The model under review builds one solid part; all positions refer to its coordinate system, in mm. A direction names the side the tool comes from. Round coordinates to 2 decimals unless told otherwise and drop trailing zeros. Write each loop counter-clockwise with the first axis right and the second up, starting at its lowest first coordinate (ties: lowest second). Pieces come first, ordered by that corner, then holes. Notation, with made-up numbers: M 56,-0.75 L 78,-0.75 A12 ccw 78,7.25 Z; hole C -1.75,52.25 d1. An arc over 180 degrees is marked long. One line per item, written item: value. Start each with the question number.
1) For P1, Ø2, axis at x = -1, z = 6, coming from the +Y side; P2, Ø1.5, axis at x = 12, z = 5, coming from the -Y side; P3, Ø2, axis at x = 5.5, z = 4, coming from the +Y side; P4, Ø3, axis at y = 6, z = 5.5, coming from the +X side, all flat-tipped, find the tip position at first contact; note any pin that passes through.
2) Take a section at D-D, the plane x = 8. Write out the cut boundary in (y, z), and give its area (3 significant figures).
3) Tool access review of faces 4 (the face through (0, 6.35, 4)), 5 (the face through (0, 7, 0)): name each direction out of +Z, -Z, +X, -X, +Y, -Y from which nothing blocks a thin tool from reaching the whole face with its end or side.
4) Take a section at B-B, the plane y = 4.5. Write out the cut boundary in (x, z), and give its area (3 significant figures).
5) Mouldability with a two-part tool opening along X and no side actions: class faces 1 (the face through (-5.474, -3.219, 3.913)), 2 (the face through (-14.274, -0.628, 3.131)), 3 (the face through (-11.83, 8.31, 6.35)) as +X half, -X half, draft (parallel to the pull), parting line (faces both ways), or undercut.
6) Wall thickness on probe 1 along Y at (x, z) = (-1.5, 6.75); probe 2 along Y at (x, z) = (-5, 7.25); probe 3 along X at (y, z) = (1.5, 2.5): over which ranges is each line inside the solid? List them lowest first.
Autodesk Inventor part; units mm, degrees
ref_plane "YZ Plane" through (0, 0, 0) normal (1, 0, 0) x (0, 1, 0)
ref_plane "XZ Plane" through (0, 0, 0) normal (0, 1, 0) x (-1, 0, 0)
ref_plane "XY Plane" through (0, 0, 0) normal (0, 0, 1) x (1, 0, 0)
sketch "Sketch1" plane through (0, 0, 0) normal (0, 0, 1) x (1, 0, 0)
  line L0 (3.6662, 6.35) -> (7.3323, 0)
  line L1 (7.3323, 0) -> (3.6662, -6.35)
  line L2 (3.6662, -6.35) -> (-3.6662, -6.35)
  line L3 (-3.6662, -6.35) -> (-7.3323, 0)
  line L4 (-7.3323, 0) -> (-3.6662, 6.35)
  line L5 (-3.6662, 6.35) -> (3.6662, 6.35)
  circle A0 centre (0, 0) radius 14.2875
  dimension "d0" = 12.7
  dimension "d1" = 28.575
extrude "Extrusion1" add sketch "Sketch1" along normal blind 6.35
sketch "Sketch2" plane through (0, 0, 6.35) normal (0, 0, 1) x (1, 0, 0)
  circle A0 centre (0, 0) radius 14.2875
  circle A1 centre (0, 0) radius 15.875
  line L0 (-3.6662, 6.35) -> (3.6662, 6.35)
  line L1 (3.6662, 6.35) -> (7.3323, 0)
  line L2 (7.3323, 0) -> (3.6662, -6.35)
  line L3 (3.6662, -6.35) -> (-3.6662, -6.35)
  line L4 (-3.6662, -6.35) -> (-7.3323, 0)
  line L5 (-7.3323, 0) -> (-3.6662, 6.35)
  line L6 (-3.6662, 6.35) -> (3.6662, 6.35)
  point P0 (0, 6.35)
  dimension "d4" = 1.5875
extrude "Extrusion2" add sketch "Sketch2" along normal blind 1.5875 contours A0 | A1
properties part number "Hex Bearing 1-2 in (FR8ZZ-Hex, am-0279)" material "Steel, Alloy"
Checked values:
1. P1: stops at y = 15.87
1. P2: stops at y = -8.81
1. P3: stops at y = 13.56
1. P4: stops at x = 15.14
2. outline: M -13.71,6.35 L -11.84,6.35 L -11.84,0 L 11.84,0 L 11.84,6.35 L 13.71,6.35 L 13.71,7.94 L -13.71,7.94 Z
2. area: 194 mm2
3. face 4: +Z, -Z
3. face 5: -Z, +X, -X, +Y, -Y
4. outline: M -15.22,6.35 L -13.56,6.35 L -13.56,0 L -4.73,0 L -4.73,7.94 L -15.22,7.94 Z; M 4.73,0 L 13.56,0 L 13.56,6.35 L 15.22,6.35 L 15.22,7.94 L 4.73,7.94 Z
4. area: 145 mm2
5. face 1: undercut
5. face 2: parting line
5. face 3: draft
6. probe 1: y = -15.8 to -6.35, 6.35 to 15.8
6. probe 2: y = -15.07 to -4.04, 4.04 to 15.07
6. probe 3: x = -14.21 to -6.47, 6.47 to 14.21
